For this review, use the dimensioned drawing (mm, ordinates from the lowest corner) and the shaded views. Round coordinates to 2 decimals unless told otherwise and drop trailing zeros. Order: outer loops, then holes, each group sorted by start corner. A loop starts at its lowest first (then second) coordinate and runs counter-clockwise, first axis right, second up. Notation, with made-up numbers: (-33, 5.5) -> (20, 5.5) arc R28 ccw to (20, 43.5) -> close; hole circle Ø10 at (-40, -17). An arc over 180 degrees is marked (long way). Answer in a Markdown table with one row per item.
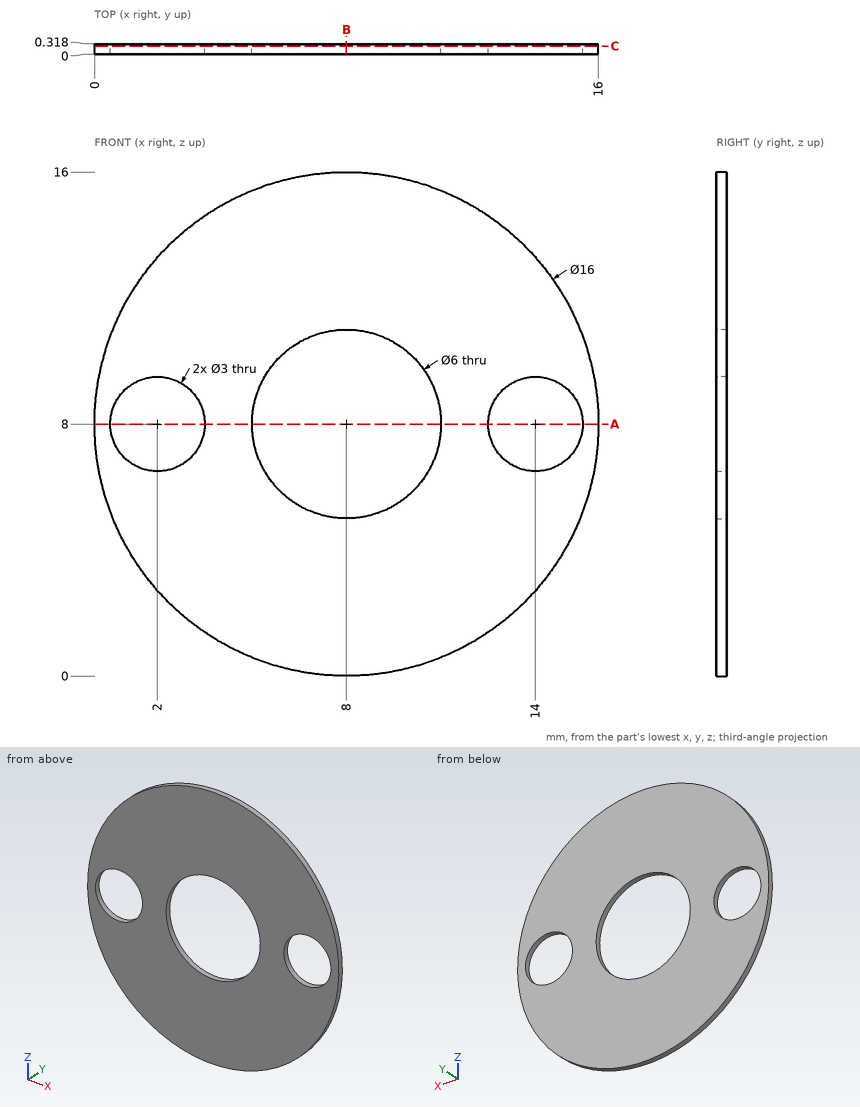
Q1. Take a section at C-C, the plane y = 0.25. Write out the cut boundary in (x, z).
Answer key:
| item | result |
|---|---|
| outline | circle Ø16 at (8, 8); hole circle Ø3 at (2, 8); hole circle Ø6 at (8, 8); hole circle Ø3 at (14, 8) |
Q2. Take a section at B-B, the plane x = 8. Write out the cut boundary in (y, z).
Answer key:
| item | result |
|---|---|
| outline | (0, 0) -> (0.32, 0) -> (0.32, 5) -> (0, 5) -> close; (0, 11) -> (0.32, 11) -> (0.32, 16) -> (0, 16) -> close |
Q3. To check wall thickness, follow probe 1 along X at (y, z) = (0.15, 8); probe 2 along X at (y, z) = (0.15, 10.5) (1 decimal); probe 3 along Z at (x, y) = (5.25, 0.15) (1 decimal). State the ranges of each line that lie inside material, in increasing order.
Answer key:
| item | result |
|---|---|
| probe 1 | x = 0 to 0.5, 3.5 to 5, 11 to 12.5, 15.5 to 16 |
| probe 2 | x = 0.4 to 6.3, 9.7 to 15.6 |
| probe 3 | z = 0.5 to 6.8, 9.2 to 15.5 |
Q4. Take a section at A-A, the plane z = 8. Write out the cut boundary in (x, y).
Answer key:
| item | result |
|---|---|
| outline | (0, 0) -> (0.5, 0) -> (0.5, 0.32) -> (0, 0.32) -> close; (3.5, 0) -> (5, 0) -> (5, 0.32) -> (3.5, 0.32) -> close; (11, 0) -> (12.5, 0) -> (12.5, 0.32) -> (11, 0.32) -> close; (15.5, 0) -> (16, 0) -> (16, 0.32) -> (15.5, 0.32) -> close |
